Autodesk Inventor part; units mm, degrees
ref_plane "YZ Plane" through (0, 0, 0) normal (1, 0, 0) x (0, 1, 0)
ref_plane "XZ Plane" through (0, 0, 0) normal (0, 1, 0) x (-1, 0, 0)
ref_plane "XY Plane" through (0, 0, 0) normal (0, 0, 1) x (1, 0, 0)
sketch "Sketch1" plane through (0, 0, 0) normal (0, 0, 1) x (1, 0, 0)
  line L0 (-15, 73) -> (15, 73)
  line L1 (15, 73) -> (15, 70)
  line L2 (-15, 70) -> (-15, 73)
  line L3 (-40.4145, 70) -> (-15, 70)
  line L4 (15, 70) -> (40.4145, 70)
  line L5 (-70.7199, 23.5096) -> (-55.7199, 49.4904)
  line L6 (-55.7199, 49.4904) -> (-53.1218, 47.9904)
  line L7 (-68.1218, 22.0096) -> (-70.7199, 23.5096)
  line L8 (-55.7199, -49.4904) -> (-70.7199, -23.5096)
  line L9 (-70.7199, -23.5096) -> (-68.1218, -22.0096)
  line L10 (-53.1218, -47.9904) -> (-55.7199, -49.4904)
  line L11 (15, -73) -> (-15, -73)
  line L12 (-15, -73) -> (-15, -70)
  line L13 (15, -70) -> (15, -73)
  line L14 (70.7199, -23.5096) -> (55.7199, -49.4904)
  line L15 (55.7199, -49.4904) -> (53.1218, -47.9904)
  line L16 (68.1218, -22.0096) -> (70.7199, -23.5096)
  line L17 (55.7199, 49.4904) -> (70.7199, 23.5096)
  line L18 (70.7199, 23.5096) -> (68.1218, 22.0096)
  line L19 (53.1218, 47.9904) -> (55.7199, 49.4904)
  line L20 (-80.829, 0) -> (-68.1218, 22.0096)
  line L21 (-53.1218, 47.9904) -> (-40.4145, 70)
  line L22 (40.4145, 70) -> (53.1218, 47.9904)
  line L23 (68.1218, 22.0096) -> (80.829, 0)
  line L24 (80.829, 0) -> (68.1218, -22.0096)
  line L25 (53.1218, -47.9904) -> (40.4145, -70)
  line L26 (40.4145, -70) -> (15, -70)
  line L27 (-15, -70) -> (-40.4145, -70)
  line L28 (-40.4145, -70) -> (-53.1218, -47.9904)
  line L29 (-68.1218, -22.0096) -> (-80.829, 0)
  line L30 (15, 70) -> (-15, 70)
  line L31 (-53.1218, 47.9904) -> (-68.1218, 22.0096)
  line L32 (-68.1218, -22.0096) -> (-53.1218, -47.9904)
  line L33 (-15, -70) -> (15, -70)
  line L34 (53.1218, -47.9904) -> (68.1218, -22.0096)
  line L35 (68.1218, 22.0096) -> (53.1218, 47.9904)
  line L36 (-15, 73) -> (-15, 79)
  line L37 (-15, 79) -> (-21, 79)
  line L38 (-21, 79) -> (-21, 70)
  line L39 (15, 73) -> (15, 79)
  line L40 (15, 79) -> (21, 79)
  line L41 (21, 79) -> (21, 70)
  line L42 (-55.7199, 49.4904) -> (-60.916, 52.4904)
  line L43 (-57.916, 57.6865) -> (-50.1218, 53.1865)
  line L44 (-60.916, 52.4904) -> (-57.916, 57.6865)
  line L45 (-70.7199, 23.5096) -> (-75.916, 26.5096)
  line L46 (-75.916, 26.5096) -> (-78.916, 21.3135)
  line L47 (-78.916, 21.3135) -> (-71.1218, 16.8135)
  line L48 (-70.7199, -23.5096) -> (-75.916, -26.5096)
  line L49 (-78.916, -21.3135) -> (-71.1218, -16.8135)
  line L50 (-75.916, -26.5096) -> (-78.916, -21.3135)
  line L51 (-55.7199, -49.4904) -> (-60.916, -52.4904)
  line L52 (-60.916, -52.4904) -> (-57.916, -57.6865)
  line L53 (-57.916, -57.6865) -> (-50.1218, -53.1865)
  line L54 (-15, -73) -> (-15, -79)
  line L55 (-21, -79) -> (-21, -70)
  line L56 (-15, -79) -> (-21, -79)
  line L57 (15, -73) -> (15, -79)
  line L58 (15, -79) -> (21, -79)
  line L59 (21, -79) -> (21, -70)
  line L60 (55.7199, -49.4904) -> (60.916, -52.4904)
  line L61 (57.916, -57.6865) -> (50.1218, -53.1865)
  line L62 (60.916, -52.4904) -> (57.916, -57.6865)
  line L63 (70.7199, -23.5096) -> (75.916, -26.5096)
  line L64 (75.916, -26.5096) -> (78.916, -21.3135)
  line L65 (78.916, -21.3135) -> (71.1218, -16.8135)
  line L66 (70.7199, 23.5096) -> (75.916, 26.5096)
  line L67 (78.916, 21.3135) -> (71.1218, 16.8135)
  line L68 (75.916, 26.5096) -> (78.916, 21.3135)
  line L69 (55.7199, 49.4904) -> (60.916, 52.4904)
  line L70 (60.916, 52.4904) -> (57.916, 57.6865)
  line L71 (57.916, 57.6865) -> (50.1218, 53.1865)
  line L72 (-21, 79) -> (-26.1962, 70)
  line L73 (21, 79) -> (26.1962, 70)
  line L74 (-57.916, 57.6865) -> (-47.5237, 57.6865)
  line L75 (-78.916, 21.3135) -> (-73.7199, 12.3135)
  line L76 (-78.916, -21.3135) -> (-73.7199, -12.3135)
  line L77 (-57.916, -57.6865) -> (-47.5237, -57.6865)
  line L78 (-21, -79) -> (-26.1962, -70)
  line L79 (21, -79) -> (26.1962, -70)
  line L80 (57.916, -57.6865) -> (47.5237, -57.6865)
  line L81 (78.916, -21.3135) -> (73.7199, -12.3135)
  line L82 (78.916, 21.3135) -> (73.7199, 12.3135)
  line L83 (57.916, 57.6865) -> (47.5237, 57.6865)
  point P0 (0, 0)
  point P1 (0, 0)
  point P2 (0, 73)
  point P3 (-63.2199, 36.5)
  point P4 (-63.2199, -36.5)
  point P5 (0, -73)
  point P6 (63.2199, -36.5)
  point P7 (63.2199, 36.5)
  point P8 (71.1218, 16.8135)
  point P9 (50.1218, -53.1865)
  point P10 (71.1218, -16.8135)
  point P11 (21, -70)
  point P12 (-71.1218, -16.8135)
  point P13 (-50.1218, -53.1865)
  point P14 (-71.1218, 16.8135)
  point P15 (-50.1218, 53.1865)
  point P16 (-47.5237, 57.6865)
  point P17 (-73.7199, 12.3135)
  point P18 (-73.7199, -12.3135)
  point P19 (-47.5237, -57.6865)
  point P20 (-26.1962, -70)
  point P21 (26.1962, -70)
  point P22 (47.5237, -57.6865)
  point P23 (73.7199, -12.3135)
  point P24 (73.7199, 12.3135)
  point P25 (47.5237, 57.6865)
  dimension "d1" = 3
  dimension "d3" = 30
  dimension "d6" = 360
  dimension "d8" = 140
  dimension "d9" = 146
  dimension "d14" = 360
  dimension "d16" = 6
  dimension "d17" = 6
  dimension "d18" = 6
  dimension "d19" = 6
  dimension "d22" = 360
  dimension "d24" = 60
  dimension "d25" = 60
  dimension "d28" = 360
extrude "Extrusion1" add sketch "Sketch1" along normal blind 3 contours L2 L3 L38 L37 L36 | L39 L40 L41 L4 L1 | L30 L4 L22 L35 L23 L24 L34 L25 L26 L33 L27 L28 L32 L29 L20 L31 L21 L3 | L3 L72 L38 | L41 L73 L4 | L21 L43 L74 | L83 L71 L22 | L21 L6 L42 L44 L43 | L71 L70 L69 L19 L22 | L20 L47 L46 L45 L7 | L18 L66 L68 L67 L23 | L20 L75 L47 | L67 L82 L23 | L29 L49 L76 | L81 L65 L24 | L29 L9 L48 L50 L49 | L65 L64 L63 L16 L24 | L28 L53 L52 L51 L10 | L15 L60 L62 L61 L25 | L28 L77 L53 | L61 L80 L25 | L27 L55 L78 | L79 L59 L26 | L27 L12 L54 L56 L55 | L59 L58 L57 L13 L26
properties material "MDF Medium Density Fiberboard"
Work out the finished part from the listing and answer in its coordinate system (mm). A direction names the side the tool comes from. Give positions to 0.01 mm unless a question says otherwise; leave off trailing zeros. Order: outer loops, then holes, each group sorted by start corner. A loop starts at its lowest first (then second) coordinate and runs counter-clockwise, first axis right, second up. Notation, with made-up numbers: (76, 83.5) - (110, 83.5) arc R21 ccw to (110, 100.5) - close; hole circle Ø4 at (-13.5, 57). An arc over 180 degrees is marked (long way). Answer as CSV lines item,"result". Start each with the question number.
Q1. The part is cut by section A-A (x = 6). Write down the section's boundary in (y, z).
Q2. The mould has two halves that part along X. Classify faces 1 (the face through (60.727, 34.818, 1.479)), 2 (the face through (-1, 1, 3)), 3 (the face through (77.324, -6.071, 1.479)): +X half, -X half, draft (parallel to the pull), parting line (faces both ways), or undercut.
Q3. Find the intervals of material crossed by L1, parallel to Y at x = 55, z = 2.75; L2, parallel to X at y = 25.5, z = 2.8; L3, parallel to Y at x = 65.5, z = 0.25, in increasing order. Write a range as [from, to].
Q4. For faces 4 (the face through (-60.727, -34.818, 1.479)), 5 (the face through (-1, 1, 0)), 6 (the face through (-77.324, 6.071, 1.479)), 7 (the face through (-23.562, 74.563, 1.479)), 8 (the face through (77.225, 6.243, 1.479)), determine the directions among +Z, -Z, +X, -X, +Y, -Y from which every point of the face is accessible in a straight line to the end or side of a thin tool.
Q5. Given pin 1 Ø0.9 at (x, z) = (-31.5, 1) entering from +Y; pin 2 Ø1.5 at (y, z) = (-73.5, 1.5) entering from +X; pin 3 Ø1.5 at (y, z) = (76.5, 2) entering from +X, each flat-ended and moving along its own axis, determine where each tip first touches the part or whether it passes through.
Q6. The part is cut by section B-B (y = -55). Write down the section's boundary in (x, z).
Check result:
1,outline,"(-70, 0) - (70, 0) - (70, 3) - (-70, 3) - close"
2,face 1,"undercut"
2,face 2,"draft"
2,face 3,"+X half"
3,L1,"y = [-57.69, -49.07], [-44.74, 44.74], [49.07, 57.69]"
3,L2,"x = [-76.5, -74.17], [-66.11, 66.11], [74.17, 76.5]"
3,L3,"y = [-26.55, 26.55]"
4,face 4,"+Z, -Z"
4,face 5,"-Z, +X, -X, +Y, -Y"
4,face 6,"+Z, -Z, -X"
4,face 7,"+Z, -Z, -X, +Y"
4,face 8,"+Z, -Z, +X"
5,pin 1,"stops at y = 70"
5,pin 2,"stops at x = 24.61"
5,pin 3,"stops at x = 22.88"
6,outline,"(-59.47, 0) - (59.47, 0) - (59.47, 3) - (-59.47, 3) - close"
